from build123d import *

# Parameters (mm, degrees)
F1_DEPTH  = 10
F3_DEPTH  = 60
F4_R      = 30
F4_R_2    = 13
F5_DEPTH  = 45
F7_DEPTH  = 10
F8_DEPTH  = 10
F9_DEPTH  = 5
F10_DEPTH = 5
F11_R     = 8.75
F12_DEPTH = 50
F13_R     = 17.5
F14_DEPTH = 1
F15_R     = 17.5
F16_DEPTH = 2


# Not quite as in the source:
# - a pattern or mirror of a feature is missing from the dataset's text; its kind, count and spacing are read off the source's solid


with BuildPart() as f1:
    # F0 (on Front) → F1 (new body, symmetric)
    with BuildSketch(Plane.XZ):
        with BuildLine():
            Line((-28.6642979162, 158.8520068331), (-70, 25))
            Line((-70, 25), (70, 25))
            Line((70, 25), (28.6642979162, 158.8520068331))
            ThreePointArc((28.6642979162, 158.8520068331), (29.6641950631, 154.4761067075), (30, 150))
            ThreePointArc((30, 150), (-4.4761067075, 120.3358049369), (-28.6642979162, 158.8520068331))
        make_face()
    extrude(amount=F1_DEPTH, both=True)

    # F2 (on Front) → F3 (join, symmetric)
    with BuildSketch(Plane.XZ):
        Polygon((70, 0), (70, 25.0431130097), (-70, 25), (-70, 0), align=None)
    extrude(amount=F3_DEPTH, both=True)

    # F4 (on Front) → F5 (join, symmetric)
    with BuildSketch(Plane.XZ):
        with Locations((0, 150)):
            Circle(F4_R)
        with Locations((0, 150)):
            Circle(F4_R_2, mode=Mode.SUBTRACT)
    extrude(amount=F5_DEPTH, both=True)

    # F6 (on Right) → F7 (join, symmetric)
    with BuildSketch(Plane.YZ):
        Polygon((60, 25), (40, 120), (10, 120), (10, 25), align=None)
    extrude(amount=F7_DEPTH, both=True)

    # F6 (on Right) → F8, piece 2 (join, symmetric)
    with BuildSketch(Plane.YZ):
        Polygon((-40, 120), (-60, 25), (-10.027478449, 25), (-10.027478449, 120), align=None)
    extrude(amount=F8_DEPTH, both=True)

    # F9 (add): a face of the model
    f9_faces = [f1.faces().sort_by_distance(p)[0] for p in [
        (5, 25, 120),
    ]]


with BuildPart() as f8:
    # F6 (on Right) → F8 (new body, symmetric)
    with BuildSketch(Plane.YZ):
        Polygon((60, 25), (40, 120), (10, 120), (10, 25), align=None)
    extrude(amount=F8_DEPTH, both=True)


with BuildPart() as f1_1:
    add(f1.part)

    add(f8.part)  # F9 merges F8
    f9 = extrude(f9_faces, amount=F9_DEPTH)

    # F9_copies: F9 across plane
    add(f9.mirror(Plane(origin=(0, 0, 0), x_dir=(0, 0, -1), z_dir=(-1, 0, 0))))

    # F10 (add): a face of the model
    f10_faces = [f1_1.faces().sort_by_distance(p)[0] for p in [
        (5, -25.0137392245, 120),
    ]]
    f10 = extrude(f10_faces, amount=F10_DEPTH)

    # F10_copies: F10 across plane
    add(f10.mirror(Plane(origin=(0, 0, 0), x_dir=(0, 0, -1), z_dir=(-1, 0, 0))))

    # F11 (on face) → F12 (cut)
    with BuildSketch(Plane(origin=(0, 0, 0), x_dir=(1, 0, 0), z_dir=(0, 0, -1))):
        with Locations((-45, -35)):
            Circle(F11_R)
        with Locations((-45, 35)):
            Circle(F11_R)
        with Locations((45, -35)):
            Circle(F11_R)
        with Locations((45, 35)):
            Circle(F11_R)
    extrude(amount=-F12_DEPTH, mode=Mode.SUBTRACT)

    # F13 (on face) → F14 (cut)
    with BuildSketch(Plane(origin=(-0.0077053893, 0, 25.021554132), x_dir=(0.9999999526, 0, 0.0003079501), z_dir=(-0.0003079501, 0, 0.9999999526))):
        with Locations((-44.992296744, -35)):
            Circle(F13_R)
        with BuildLine():
            add(Edge.make_bspline(
                [(-36.2422963292, -35), (-36.2422963292, -19.8445554338), (-49.3672969515, -27.4222777169), (-62.4922975738, -35), (-49.3672969515, -42.5777222831), (-36.2422963292, -50.1554445662), (-36.2422963292, -35)],
                knots=[3.1415926536, 3.1415926536, 3.1415926536, 5.235987756, 5.235987756, 7.3303828584, 7.3303828584, 9.4247779608, 9.4247779608, 9.4247779608], degree=2, weights=[1, 0.5, 1, 0.5, 1, 0.5, 1]))
        make_face(mode=Mode.SUBTRACT)
        with BuildLine():
            add(Edge.make_bspline(
                [(53.7577079383, -35), (53.7577079383, -19.8445554338), (40.632707316, -27.4222777169), (27.5077066937, -35), (40.632707316, -42.5777222831), (53.7577079383, -50.1554445662), (53.7577079383, -35)],
                knots=[3.1415926536, 3.1415926536, 3.1415926536, 5.235987756, 5.235987756, 7.3303828584, 7.3303828584, 9.4247779608, 9.4247779608, 9.4247779608], degree=2, weights=[1, 0.5, 1, 0.5, 1, 0.5, 1]))
        make_face()
        with BuildLine():
            add(Edge.make_bspline(
                [(-36.2422963292, -35), (-36.2422963292, -19.8445554338), (-49.3672969515, -27.4222777169), (-62.4922975738, -35), (-49.3672969515, -42.5777222831), (-36.2422963292, -50.1554445662), (-36.2422963292, -35)],
                knots=[3.1415926536, 3.1415926536, 3.1415926536, 5.235987756, 5.235987756, 7.3303828584, 7.3303828584, 9.4247779608, 9.4247779608, 9.4247779608], degree=2, weights=[1, 0.5, 1, 0.5, 1, 0.5, 1]))
        make_face()
    extrude(amount=-F14_DEPTH, mode=Mode.SUBTRACT)

    # F15 (on face) → F16 (cut)
    with BuildSketch(Plane(origin=(-0.0077053893, 0, 25.021554132), x_dir=(0.9999999526, 0, 0.0003079501), z_dir=(-0.0003079501, 0, 0.9999999526))):
        with Locations((45.0077075234, -35)):
            Circle(F15_R)
        with BuildLine():
            add(Edge.make_bspline(
                [(53.7577079383, -35), (53.7577079383, -19.8445554338), (40.632707316, -27.4222777169), (27.5077066937, -35), (40.632707316, -42.5777222831), (53.7577079383, -50.1554445662), (53.7577079383, -35)],
                knots=[3.1415926536, 3.1415926536, 3.1415926536, 5.235987756, 5.235987756, 7.3303828584, 7.3303828584, 9.4247779608, 9.4247779608, 9.4247779608], degree=2, weights=[1, 0.5, 1, 0.5, 1, 0.5, 1]))
        make_face(mode=Mode.SUBTRACT)
        with BuildLine():
            add(Edge.make_bspline(
                [(53.7577079383, -35), (53.7577079383, -19.8445554338), (40.632707316, -27.4222777169), (27.5077066937, -35), (40.632707316, -42.5777222831), (53.7577079383, -50.1554445662), (53.7577079383, -35)],
                knots=[3.1415926536, 3.1415926536, 3.1415926536, 5.235987756, 5.235987756, 7.3303828584, 7.3303828584, 9.4247779608, 9.4247779608, 9.4247779608], degree=2, weights=[1, 0.5, 1, 0.5, 1, 0.5, 1]))
        make_face()
    extrude(amount=-F16_DEPTH, mode=Mode.SUBTRACT)


solid = f1_1.part
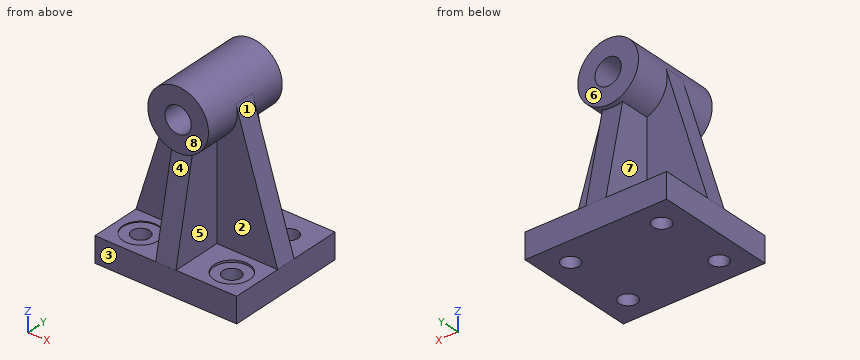
Verification items for the finished model (mm, model axes). Face numbers are marked on the shaded views. A direction names the side the tool comes from. Give positions to 0.01 mm unless a question says otherwise; leave off trailing zeros. Order: outer loops, then holes, each group sorted by start corner. A loop starts at its lowest first (then second) coordinate and runs counter-clockwise, first axis right, second up. Notation, with made-up numbers: M 73,-5 L 93,-5 A25 cw 93,21 Z; hole C -34,5.5 d5. An arc over 180 degrees is marked long. Answer as a JSON object with one key per item and string values. Group by question number.
1) Cross-section at C-C (z = 104). Enter the section's corners in (x, y).
2) Cross-section at D-D (y = 14). Enter the section's corners in (x, z), then the cut area to 3 significant figures.
3) Depth check by flat-ended pin: pin 1 Ø3 at (x, y) = (18, -19.5) entering from +Z; pin 2 Ø3 at (y, z) = (-24, 112.5) entering from -X; pin 3 Ø1.4 at (x, z) = (-6, 120.5) entering from -Y; pin 4 Ø12 at (x, y) = (27.5, 22) entering from -Z. Enter the tip coordinate at first touch or a pass-through.
4) Mould release check, pull along Y, two halves, no side actions. Record for the marked faces 1, 2 and 3: released by +Y, released by -Y, zero draft, split by the parting line, or undercut.
5) Cross-section at B-B (y = 35). Enter the section's corners in (x, z) (3 decimals).
6) Access from +Z, -Z, +X, -X, +Y, -Y to the whole of each face (thin tool, end or side, straight path). Record for the marked faces 4, 5, 6, 7 and 8.
7) Scan lines: line 1 along Y through (x, z) = (-45, 7); line 2 along X through (y, z) = (-35, 8.5); line 3 along Y through (x, z) = (-45, 24.7). Record each from-to range of solid material in increasing order. Write a range as [from, to].
Result sheet:
{
 "1": {"outline": "M -45.6,-10 L 45.6,-10 L 45.6,10 L 10,10 L 10,43.37 L -10,43.37 L -10,10 L -45.6,10 Z; M -10,-43.37 L 10,-43.37 L 10,-10.03 L -10,-10.03 Z"},
 "2": {"outline": "M -70,0 L 70,0 L 70,25.04 L 10,25.02 L 10,121.72 A30 ccw long -10,121.72 L -10,25.02 L -70,25 Z; hole C 0,150 d26", "area": "7,710 mm2"},
 "3": {"pin 1": "stops at z = 175.05", "pin 2": "stops at x = -10", "pin 3": "stops at y = -45", "pin 4": "stops at z = 0"},
 "4": {"face 1": "zero draft", "face 2": "undercut", "face 3": "released by -Y"},
 "5": {"outline": "M -70,0 L -53.75,0 L -53.75,25.005 L -70,25 Z; M -36.25,0 L 36.25,0 L 36.25,25.033 L 10,25.025 L 10,121.716 A30 ccw long -10,121.716 L -10,25.018 L -36.25,25.01 Z; M 53.75,0 L 70,0 L 70,25.043 L 53.75,25.038 Z; hole C 0,150 d26"},
 "6": {"face 4": "+X, -X, -Y", "face 5": "+X, -Y", "face 6": "+Z, +X, -X, +Y", "face 7": "-X, +Y", "face 8": "+Z, +X, -X, -Y"},
 "7": {"line 1": "y = [-60, -43.75], [-26.25, 26.25], [43.75, 60]", "line 2": "x = [-70, -53.75], [-36.25, 36.25], [53.75, 70]", "line 3": "y = [-60, -52.5], [-17.5, 26.25], [43.75, 60]"}
}
